Build history of the part. All positions in model axes, mm. Face numbers are marked on the shaded views. A direction names the side the tool comes from. Give positions to 0.01 mm unless a question says otherwise; leave off trailing zeros. Order: outer loops, then holes, each group sorted by start corner. A loop starts at its lowest first (then second) coordinate and runs counter-clockwise, first axis right, second up. Notation, with made-up numbers: (60, 75) -> (82, 75) arc R17 cw to (82, 86) -> close; hole circle Ø6 at (56.25, -19). An arc over 180 degrees is marked (long way). One line per question, with ' | ' between items. Start each with the question number.
(1) Pin check, flat tip, straight feed: pin 1 Ø17 at (x, z) = (0, 0) entering from -Y. Stop position of the tip, or through.
(2) Cut at D-D (z = 59.5). Give the cut face in (x, y).
(3) Cut at B-B (x = 0). Give the cut face in (y, z), then the cut area to 3 significant figures.
(4) Drill centre lines: L1, parallel to Y at x = 58.5, z = 0; L2, parallel to Z at x = 0, y = -5; L3, parallel to Z at x = 0, y = -79.5. Where is each one in solid material? Low to high. Write a range as from..to.
(5) Cut at A-A (z = 0). Give the cut face in (x, y).
(6) Cut at C-C (y = -76). Give the cut face in (x, z).
(7) Which spindle directions (+Z, -Z, +X, -X, +Y, -Y) get a long thin tool onto all of the face, cutting with end or side? Do the marked faces 1 and 2. Say none if no direction does.
from build123d import *

# Parameters (mm, degrees)
F0_R     = 100
F1_DEPTH = 15
F2_R     = 16
F3_DEPTH = 150
F4_T     = -2


with BuildPart() as f1:
    # F0 (on Front) → F1 (new body)
    with BuildSketch(Plane.XZ):
        Circle(F0_R)
    extrude(amount=F1_DEPTH)

    # F2 (on face) → F3 (join)
    with BuildSketch(Plane.XZ.offset(15)):
        Circle(F2_R)
    extrude(amount=F3_DEPTH)

    # F4
    f4_openings = [f1.faces().sort_by_distance(p)[0] for p in [
        (0, -165, 0),
    ]]
    offset(amount=F4_T, openings=f4_openings, kind=Kind.INTERSECTION)


solid = f1.part
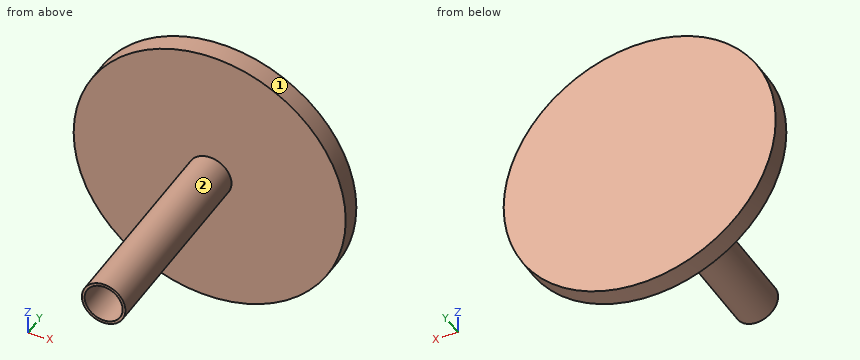
Result set:
1) pin 1: stops at y = -2
2) outline: (-80.37, -15) -> (80.37, -15) -> (80.37, 0) -> (-80.37, 0) -> close; hole (-77.87, -13) -> (77.87, -13) -> (77.87, -2) -> (-77.87, -2) -> close
3) outline: (-165, -16) -> (-15, -16) -> (-15, -100) -> (0, -100) -> (0, 100) -> (-15, 100) -> (-15, 16) -> (-165, 16) -> (-165, 14) -> (-13, 14) -> (-13, 98) -> (-2, 98) -> (-2, -98) -> (-13, -98) -> (-13, -14) -> (-165, -14) -> close | area: 1,390 mm2
4) L1: y = -15..-13, -2..0 | L2: z = -100..-98, 98..100 | L3: z = -16..-14, 14..16
5) outline: (-100, -15) -> (-16, -15) -> (-16, -165) -> (-14, -165) -> (-14, -13) -> (-98, -13) -> (-98, -2) -> (98, -2) -> (98, -13) -> (14, -13) -> (14, -165) -> (16, -165) -> (16, -15) -> (100, -15) -> (100, 0) -> (-100, 0) -> close
6) outline: circle Ø32 at (0, 0); hole circle Ø28 at (0, 0)
7) face 1: +Y, -Y | face 2: -Y
